Autodesk Inventor part; units mm, degrees
ref_plane "YZ Plane" through (0, 0, 0) normal (1, 0, 0) x (0, 1, 0)
ref_plane "XZ Plane" through (0, 0, 0) normal (0, 1, 0) x (-1, 0, 0)
ref_plane "XY Plane" through (0, 0, 0) normal (0, 0, 1) x (1, 0, 0)
sketch "Esquisse1" plane through (0, 0, 0) normal (0, 1, 0) x (-1, 0, 0)
  line L0 (0, 0) -> (85, 0)
  line L1 (85, 0) -> (85, 50)
  line L2 (85, 50) -> (0, 50)
  line L3 (0, 50) -> (0, 0)
  dimension "d0" = 85
  dimension "d1" = 50
extrude "Extrusion1" add sketch "Esquisse1" along normal blind 27
sketch "Esquisse2" plane through (0, 27, 0) normal (0, 1, 0) x (1, 0, 0)
  line L0 (0, 0) -> (-85, 0)
  line L1 (-85, 0) -> (-85, -50)
  line L2 (-85, -50) -> (0, -50)
  line L3 (0, -50) -> (0, 0)
  line L4 (-82.5, -2.5) -> (-78.5532, -2.5)
  line L5 (-2.5, -2.5) -> (-2.5, -5.8909)
  line L6 (-2.5, -47.5) -> (-78.5532, -47.5)
  line L7 (-82.5, -47.5) -> (-82.5, -44.1091)
  line L8 (-82.5, -2.5) -> (-2.5, -47.5) construction
  line L9 (-2.5, -2.5) -> (-82.5, -47.5) construction
  circle A0 centre (-81.5, -3.0625) radius 2
  arc A1 (-78.8853, -4.5333) -> (-78.5532, -2.5) centre (-81.5, -3.0625) ccw
  line L10 (-42.5, -25) -> (-42.5, -2.5) construction
  line L11 (-42.5, -25) -> (-82.5, -25) construction
  circle A2 centre (-3.5, -3.0625) radius 2
  arc A3 (-6.1147, -4.5333) -> (-2.5, -5.8909) centre (-3.5, -3.0625) ccw
  circle A4 centre (-81.5, -46.9375) radius 2
  arc A5 (-78.5532, -47.5) -> (-82.5, -44.1091) centre (-81.5, -46.9375) ccw
  circle A6 centre (-3.5, -46.9375) radius 2
  arc A7 (-6.1147, -45.4667) -> (-6.4468, -47.5) centre (-3.5, -46.9375) ccw
  arc A8 (-82.5, -5.8909) -> (-78.8853, -4.5333) centre (-81.5, -3.0625) ccw
  arc A9 (-78.5532, -2.5) -> (-82.5, -5.8909) centre (-81.5, -3.0625) ccw
  arc A10 (-6.4468, -2.5) -> (-6.1147, -4.5333) centre (-3.5, -3.0625) ccw
  arc A11 (-2.5, -5.8909) -> (-6.4468, -2.5) centre (-3.5, -3.0625) ccw
  arc A12 (-2.5, -44.1091) -> (-6.1147, -45.4667) centre (-3.5, -46.9375) ccw
  arc A13 (-6.4468, -47.5) -> (-2.5, -44.1091) centre (-3.5, -46.9375) ccw
  arc A14 (-82.5, -44.1091) -> (-78.5532, -47.5) centre (-81.5, -46.9375) ccw
  line L12 (-78.5532, -47.5) -> (-82.5, -47.5)
  line L13 (-82.5, -44.1091) -> (-82.5, -2.5)
  line L14 (-42.5, -2.5) -> (-6.4468, -2.5)
  line L15 (-78.5532, -2.5) -> (-42.5, -2.5)
  line L16 (-6.4468, -2.5) -> (-2.5, -2.5)
  line L17 (-2.5, -5.8909) -> (-2.5, -25)
  line L18 (-2.5, -44.1091) -> (-2.5, -47.5)
  line L19 (-2.5, -25) -> (-2.5, -44.1091)
  dimension "d4" = 2.5
  dimension "d5" = 2.5
  dimension "d6" = 2.5
  dimension "d7" = 2.5
  dimension "d8" = 4
  dimension "d9" = 6
  dimension "d10" = 1
extrude "Extrusion2" cut sketch "Esquisse2" against normal blind 25 contours L13 A0 L4 | L4 A0 L13 | L15 L14 A10 A3 L17 L19 A12 A7 L6 A5 L13 A8 A1 | A4 L12 L7 | L7 L12 A4 | L16 L5 A2 | A2 L5 L16 | A6 L18 L6 | L6 L18 A6
equation "\"d5\" = d4"
equation "\"d6\" = d4"
equation "\"d7\" = d4"
properties part number "conrad_Strapubox_2028"
Model file for the job. Use its own axes, mm. A direction names the side the tool comes from. Round coordinates to 2 decimals unless told otherwise and drop trailing zeros. Write each loop counter-clockwise with the first axis right and the second up, starting at its lowest first coordinate (ties: lowest second). Pieces come first, ordered by that corner, then holes. Notation, with made-up numbers: M -5,46 L 30,46 A15 cw 30,75 Z; hole C 72,44.5 d4. An arc over 180 degrees is marked long. Put each result on its own line as item: value.
Item 1: Cut at C-C (x = -3.5). List the corners of the cut face in (y, z), and give its area (3 significant figures).
Responses:
outline: M 0,0 L 27,0 L 27,1.06 L 2,1.06 L 2,5.06 L 27,5.06 L 27,6.06 L 2,6.06 L 2,43.94 L 27,43.94 L 27,44.94 L 2,44.94 L 2,48.94 L 27,48.94 L 27,50 L 0,50 Z
area: 203 mm²
Item 2: Flat gauge pin, fed straight in: P1, Ø2, axis at x = -82, z = 2.5, coming from the +Y side. Where does the tip first touch, or does it go through?
Responses:
P1: y = 2
Item 3: Probe L1, parallel to Z at x = -81.5, y = 18; L2, parallel to X at y = 13, z = 7.5; L3, parallel to Z at x = -9, y = 20.25. List the from-to ranges inside material, lowest first. Write a range as from..to.
Responses:
L1: 0..1.06, 5.06..6.06, 43.94..44.94, 48.94..50
L2: -85..-82.5, -2.5..0
L3: 0..2.5, 47.5..50
Item 4: Mould opens along Z. For faces 3 (the flat face through (-42, 13, 0)), 4 (the cylindrical face through (-4, 15, 5)), 5 (the flat face through (0, 13, 25)) say: +Z half, -Z half, draft (parallel to the pull), parting line (faces both ways), or undercut.
Responses:
face 3: -Z half
face 4: undercut
face 5: draft
Item 5: Tool access for faces 1 (the flat face through (-2.5, 15, 25)), 2 (the flat face through (-42, 0, 25)): list every direction of +Z, -Z, +X, -X, +Y, -Y with a clear straight run to the whole face (end or side of a thin tool).
Responses:
face 1: +Y
face 2: +Z, -Z, +X, -X, -Y
Item 6: Cut at B-B (z = 38). List the corners of the cut face in (x, y), and give its area (3 significant figures).
Responses:
outline: M -85,0 L 0,0 L 0,27 L -2.5,27 L -2.5,2 L -82.5,2 L -82.5,27 L -85,27 Z
area: 295 mm²
Item 7: Cut at A-A (x = -47). List the corners of the cut face in (y, z), and give its area (3 significant figures).
Responses:
outline: M 0,0 L 27,0 L 27,2.5 L 2,2.5 L 2,47.5 L 27,47.5 L 27,50 L 0,50 Z
area: 225 mm²
